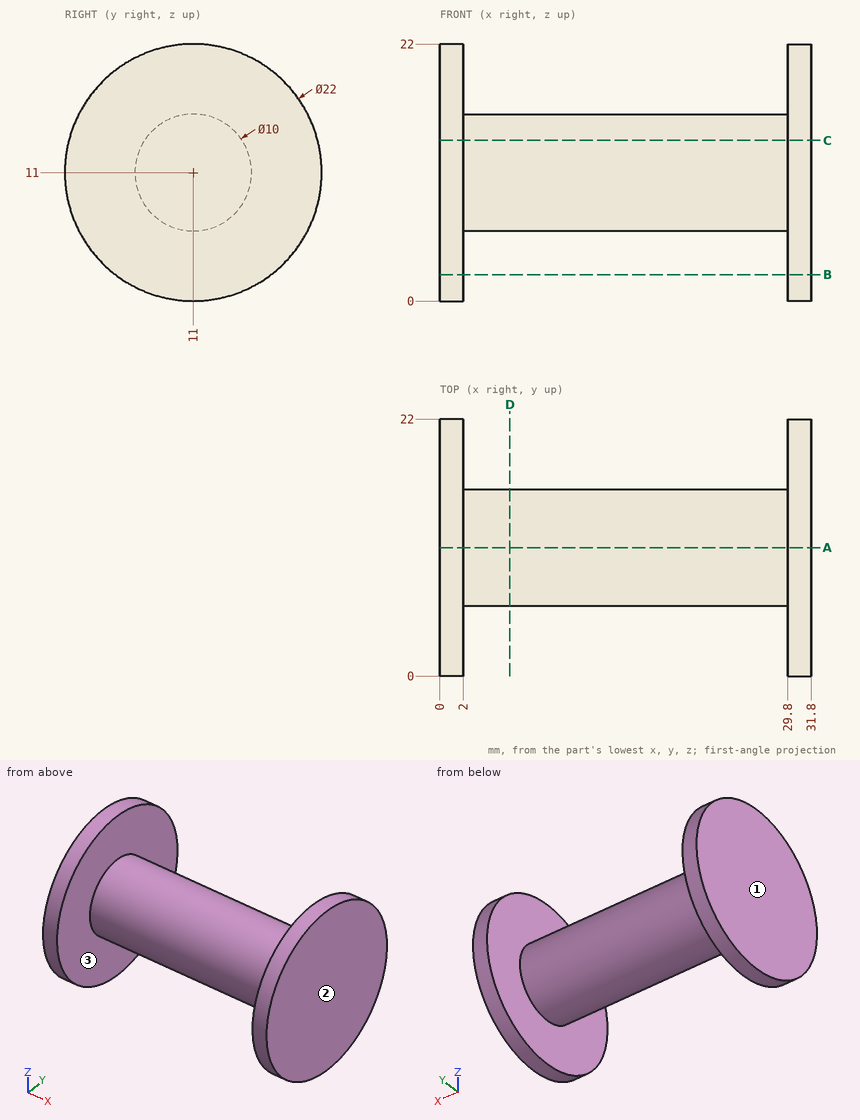
For this review, use the dimensioned drawing (mm, ordinates from the lowest corner) and the shaded views. Give positions to 0.01 mm unless a question says otherwise; leave off trailing zeros. Order: outer loops, then holes, each group sorted by start corner. A loop starts at its lowest first (then second) coordinate and runs counter-clockwise, first axis right, second up.
1) Wall thickness on line 1 (X direction, y = 9, z = 19.75); line 2 (Y direction, x = 22, z = 8.5); line 3 (Y direction, x = 21.5, z = 14): over which ranges is each line inside the solid? List them lowest first.
2) Take a section at B-B (z = 2.25). Give the boundary of the cut face in (x, y).
3) Take a section at A-A (y = 11). Give the boundary of the cut face in (x, z), then the cut area to 3 significant figures.
4) Take a section at D-D (x = 6). Give the boundary of the cut face in (y, z), then the cut area to 3 significant figures.
5) Insertion check: pin 1 (8 mm diameter, centred on x = 9.5, y = 14, fed in from +Z); pin 2 (12 mm diameter, centred on x = 28, y = 15.5, fed in from +Z); pin 3 (12 mm diameter, centred on x = 13.5, z = 18.5, fed in from -Y). Each pin has a flat end and moves straight along its axis. Give the tip position at first contact, or say it passes through.
6) The part is to be moulded in two halves that separate along X. For the marked faces 1, 2 and 3, say which applies: released by +X, released by -X, zero draft, split by the parting line, or undercut.
7) Take a section at C-C (z = 13.75). Give the boundary of the cut face in (x, y).
Derived:
1. line 1: x = 0 to 2, 29.8 to 31.8
1. line 2: y = 6.67 to 15.33
1. line 3: y = 7 to 15
2. outline: (0, 4.33) - (2, 4.33) - (2, 17.67) - (0, 17.67) - close; (29.8, 4.33) - (31.8, 4.33) - (31.8, 17.67) - (29.8, 17.67) - close
3. outline: (0, 0) - (2, 0) - (2, 6) - (29.8, 6) - (29.8, 0) - (31.8, 0) - (31.8, 22) - (29.8, 22) - (29.8, 16) - (2, 16) - (2, 22) - (0, 22) - close
3. area: 366 mm2
4. outline: circle Ø10 at (11, 11)
4. area: 78.5 mm2
5. pin 1: stops at z = 16
5. pin 2: stops at z = 22
5. pin 3: stops at y = 6.23
6. face 1: released by -X
6. face 2: released by +X
6. face 3: undercut
7. outline: (0, 0.35) - (2, 0.35) - (2, 6.82) - (29.8, 6.82) - (29.8, 0.35) - (31.8, 0.35) - (31.8, 21.65) - (29.8, 21.65) - (29.8, 15.18) - (2, 15.18) - (2, 21.65) - (0, 21.65) - close
